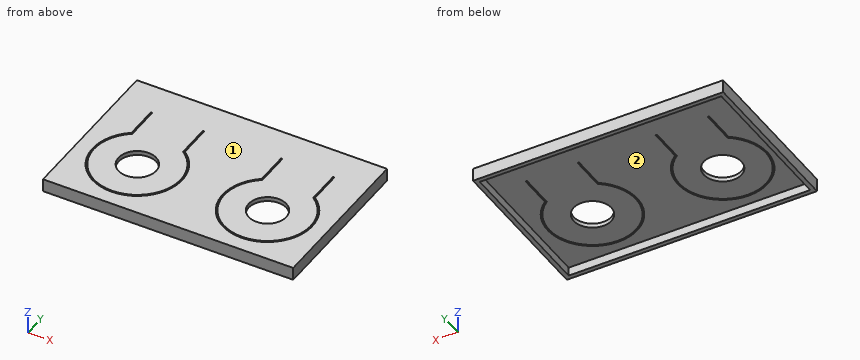
```python
from build123d import *

# Parameters (mm, degrees)
SKETCH002_W           = 173
SKETCH002_H           = 112
SKETCH002_W_2         = 167
SKETCH002_H_2         = 106
EXTRUDE001_DEPTH      = 3
EXTRUDE001_DEPTH_BACK = 6
SKETCH_W              = 167
SKETCH_H              = 106
SKETCH_R              = 13
EXTRUDE_DEPTH         = 3


with BuildPart() as notch:
    # Sketch002 → Extrude001 (new body, two sides)
    with BuildSketch(Plane.XY) as extrude001_sk:
        Rectangle(SKETCH002_W, SKETCH002_H)
        Rectangle(SKETCH002_W_2, SKETCH002_H_2, mode=Mode.SUBTRACT)
    extrude(amount=EXTRUDE001_DEPTH)
    extrude(extrude001_sk.sketch, amount=-EXTRUDE001_DEPTH_BACK)


with BuildPart() as lid:
    # Sketch → Extrude (new body)
    with BuildSketch(Plane.XY):
        Rectangle(SKETCH_W, SKETCH_H)
        with Locations((-45, -15)):
            Circle(SKETCH_R, mode=Mode.SUBTRACT)
        with Locations((45, -15)):
            Circle(SKETCH_R, mode=Mode.SUBTRACT)
        with BuildLine():
            Line((-27.5, 9.366986), (-27.5, 33))
            Line((-27.5, 33), (-26.5, 33))
            Line((-26.5, 33), (-26.5, 9.874686))
            ThreePointArc((-63.5, 9.874686), (-45, -46), (-26.5, 9.874686))
            Line((-63.5, 9.874686), (-63.5, 33))
            Line((-63.5, 33), (-62.5, 33))
            Line((-62.5, 33), (-62.5, 9.366986))
            ThreePointArc((-62.5, 9.366986), (-45, -45), (-27.5, 9.366986))
        make_face(mode=Mode.SUBTRACT)
        with BuildLine():
            Line((27.5, 9.366986), (27.5, 33))
            Line((27.5, 33), (26.5, 33))
            Line((26.5, 33), (26.5, 9.874686))
            ThreePointArc((26.5, 9.874686), (45, -46), (63.5, 9.874686))
            Line((63.5, 9.874686), (63.5, 33))
            Line((63.5, 33), (62.5, 33))
            Line((62.5, 33), (62.5, 9.366986))
            ThreePointArc((27.5, 9.366986), (45, -45), (62.5, 9.366986))
        make_face(mode=Mode.SUBTRACT)
    extrude(amount=EXTRUDE_DEPTH)

    # Fusion001: union Notch
    add(notch.part)


solid = lid.part
```
Can you work these out from the model? Positions are in its coordinate system, mm. Face numbers are marked on the shaded views. Round coordinates to 2 decimals unless told otherwise and drop trailing zeros. Loops run counter-clockwise (first coordinate to the right, second up) from the corner with the lowest first, then second, coordinate; pieces in that order, holes last. Notation, with made-up numbers: (-28, -28) -> (-9, -28) arc R30 ccw to (-9, 7) -> close; hole circle Ø10 at (53, -32.5). An arc over 180 degrees is marked (long way). One line per item, written item: value. Start each with the question number.
1. If we mould it in two halves opening along X, with no side actions, what happens to the marked faces 1 and 2? For each: pulls with the +X half, pulls with the -X half, needs draft (parallel to the pull), parting line crosses it, or undercut.
2. If we section it at B-B, the plane x = 45: Write out the boundary of the cut face in (y, z), then the cut area to 3 significant figures.
3. For pin 1 (5 mm diameter, centred on x = -39.5, y = -26, fed in from -Z), with a flat end and sliding along its axis, tell me the tip position at first contact or that it passes through.
4. If I drill on probe 1 along X at (y, z) = (26.5, 0.75); probe 2 along X at (y, z) = (-6, -0.5); probe 3 along Y at (x, z) = (-4.5, -2.75), over which ranges is the centre line in solid material (lowest first)?
5. If we section it at C-C, the plane z = -3: Write out the boundary of the cut face in (x, y).
6. If we section it at D-D, the plane y = -15: Give the number of separate pieces and of enclosed holes in the cut face, then the cut area to 3 significant figures.
7. If we section it at A-A, the plane y = 21.5: Write out the boundary of the cut face in (x, z).
Calculated:
1. face 1: needs draft
1. face 2: undercut
2. outline: (-56, -6) -> (-53, -6) -> (-53, 0) -> (-46, 0) -> (-46, 3) -> (-56, 3) -> close; (-45, 0) -> (-28, 0) -> (-28, 3) -> (-45, 3) -> close; (-2, 0) -> (53, 0) -> (53, -6) -> (56, -6) -> (56, 3) -> (-2, 3) -> close
2. area: 291 mm²
3. pin 1: stops at z = 0
4. probe 1: x = -86.5 to -63.5, -62.5 to -27.5, -26.5 to 26.5, 27.5 to 62.5, 63.5 to 86.5
4. probe 2: x = -86.5 to -83.5, 83.5 to 86.5
4. probe 3: y = -56 to -53, 53 to 56
5. outline: (-86.5, -56) -> (86.5, -56) -> (86.5, 56) -> (-86.5, 56) -> close; hole (-83.5, -53) -> (83.5, -53) -> (83.5, 53) -> (-83.5, 53) -> close
6. separate pieces: 7
6. enclosed holes: 0
6. area: 387 mm²
7. outline: (-86.5, -6) -> (-83.5, -6) -> (-83.5, 0) -> (-63.5, 0) -> (-63.5, 3) -> (-86.5, 3) -> close; (-62.5, 0) -> (-27.5, 0) -> (-27.5, 3) -> (-62.5, 3) -> close; (-26.5, 0) -> (26.5, 0) -> (26.5, 3) -> (-26.5, 3) -> close; (27.5, 0) -> (62.5, 0) -> (62.5, 3) -> (27.5, 3) -> close; (63.5, 0) -> (83.5, 0) -> (83.5, -6) -> (86.5, -6) -> (86.5, 3) -> (63.5, 3) -> close
